Can you work these out from the model? Positions are in its coordinate system, mm. Face numbers are marked on the shaded views. A direction names the side the tool comes from. Coordinates: 2 decimals unless noted, no trailing zeros. Loops run counter-clockwise (first coordinate to the right, second up) from the corner with the lowest first, then second, coordinate; pieces in that order, holes last.
```python
from build123d import *

# Parameters (mm, degrees)
F1_DEPTH = 38.1
F2_W     = 25.103066
F2_H     = 7.577248
F3_DEPTH = 25.4
F4_W     = 9.944637
F4_H     = 5.652566
F5_DEPTH = 228.6
F6_R     = 5.456635
F6_R_2   = 5.70769
F6_R_3   = 5.555233
F6_R_4   = 5.475629
F7_DEPTH = 101.6


with BuildPart() as f1:
    # F0 (on Front) → F1 (new body)
    with BuildSketch(Plane.XZ):
        Polygon((0, 17.413402), (-40.967319, 17.413402), (-40.967319, -9.164948), (-8.523404, -9.164948), (-8.523404, -17.413402), (40.967319, -17.413402), align=None)
    extrude(amount=-F1_DEPTH)

    # F2 (on face) → F3 (cut)
    with BuildSketch(Plane(origin=(0, 0, -17.413402), x_dir=(1, 0, 0), z_dir=(0, 0, -1))):
        with Locations((28.415786, -3.788624)):
            Rectangle(F2_W, F2_H)
    extrude(amount=-F3_DEPTH, mode=Mode.SUBTRACT)

    # F4 (on face) → F5 (cut)
    with BuildSketch(Plane(origin=(-40.967319, 0, 0), x_dir=(0, -1, 0), z_dir=(-1, 0, 0))):
        with Locations((-19.910272, 14.587119)):
            Rectangle(F4_W, F4_H)
    extrude(amount=-F5_DEPTH, mode=Mode.SUBTRACT)

    # F6 (on face) → F7 (cut)
    with BuildSketch(Plane(origin=(0, 0, -17.413402), x_dir=(1, 0, 0), z_dir=(0, 0, -1))):
        with Locations((32.08825, -29.554859)):
            Circle(F6_R)
        with Locations((19.997094, -30.228976)):
            Circle(F6_R_2)
        with Locations((20.558245, -16.475564)):
            Circle(F6_R_3)
        with Locations((33.392582, -16.614418)):
            Circle(F6_R_4)
    extrude(amount=-F7_DEPTH, mode=Mode.SUBTRACT)


solid = f1.part
```
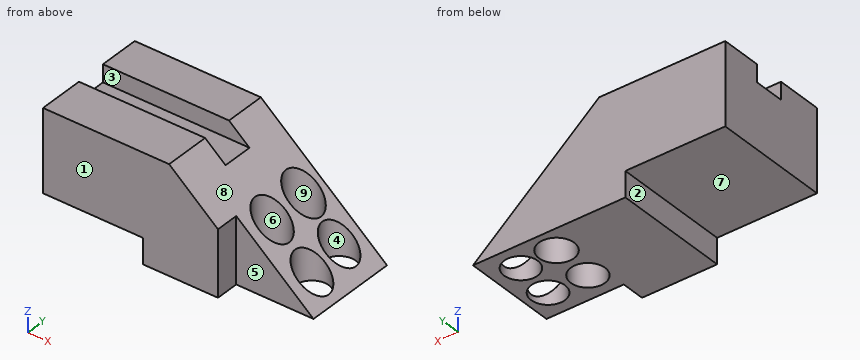
Item 1: Suppose I cut it at D-D, the plane y = 6.5. Please give me the cut outline in (x, z).
Results are:
outline: (-40.97, -9.16) - (-8.52, -9.16) - (-8.52, -17.41) - (15.86, -17.41) - (15.86, 3.93) - (0, 17.41) - (-40.97, 17.41) - close
Item 2: Suppose I cut it at C-C, the plane z = -12.5. Please give me the cut outline in (x, y), plus the area to 3 significant figures.
Results are:
outline: (-8.52, 0) - (15.86, 0) - (15.86, 7.58) - (35.19, 7.58) - (35.19, 11.44) arc R5.48 cw (long way) to (35.19, 21.79) - (35.19, 25.06) arc R5.46 cw (long way) to (35.19, 34.05) - (35.19, 38.1) - (-8.52, 38.1) - close; hole circle Ø11.42 at (20, 30.23); hole circle Ø11.11 at (20.56, 16.48)
area: 1,170 mm2
Item 3: I'm going to push flat-ended pins straight in: P1, Ø6, axis at y = 4.5, z = 13.5, coming from the +X side; P2, Ø8, axis at x = -18.5, y = 20.5, coming from the +Z side; P3, Ø10, axis at x = 20.56, y = 16.48, coming from the +Z side; P4, Ø6.5, axis at y = 21, z = -12.5, coming from the -X side. Where does each tip first touch, or does it pass through?
Results are:
P1: stops at x = 8.13
P2: stops at z = 11.76
P3: passes through
P4: stops at x = -8.52
Item 4: On a 3-axis mill with a long thin cutter (end or side, diameter ignored), from which of +Z, -Z, +X, -X, +Y, -Y can I reach the whole of each face in a straight line? I mean the marked faces 1, 2, 3, 4 and 5. Say none if no direction works.
Results are:
face 1: +Z, -Z, +X, -X, -Y
face 2: -Z, -X, +Y, -Y
face 3: +Z, +X, -X
face 4: +Z, -Z
face 5: +Z, -Z, +X, -Y
Item 5: Suppose I cut it at A-A, the plane y = 12.5. Please give me the cut outline in (x, z).
Results are:
outline: (-40.97, -9.16) - (-8.52, -9.16) - (-8.52, -17.41) - (16.68, -17.41) - (16.68, 3.24) - (0, 17.41) - (-40.97, 17.41) - close; (24.44, -17.41) - (29.78, -17.41) - (29.78, -7.9) - (24.44, -3.36) - close; (37.01, -17.41) - (40.97, -17.41) - (37.01, -14.05) - close
Item 6: We'd pull the mould along X, two halves only. Please class the marked faces 6, 7, 8 and 9: +X half, -X half, draft (parallel to the pull), parting line (faces both ways), or undercut.
Results are:
face 6: undercut
face 7: draft
face 8: +X half
face 9: undercut
Item 7: Suppose I cut it at B-B, the plane x = -35. Please give me the cut outline in (y, z), plus the area to 3 significant figures.
Results are:
outline: (0, -9.16) - (38.1, -9.16) - (38.1, 17.41) - (24.88, 17.41) - (24.88, 11.76) - (14.94, 11.76) - (14.94, 17.41) - (0, 17.41) - close
area: 956 mm2
Item 8: I need wall thicknesses on line 1 along Y through (x, z) = (-27, 13); line 2 along Z through (x, y) = (-6, 19.5); line 3 along X through (y, z) = (6, 2). Which ranges of each line are inside material? Lowest first, please.
Results are:
line 1: y = 0 to 14.94, 24.88 to 38.1
line 2: z = -17.41 to 11.76
line 3: x = -40.97 to 15.86
